Can you work these out from the drawing? Everything is in mm from the part's minimum corner. A direction names the side the tool comes from. Round coordinates to 2 decimals unless told otherwise and drop trailing zeros. Loops run counter-clockwise (first coordinate to the right, second up) from the corner with the lowest first, then second, coordinate; pieces in that order, holes last. Notation, with made-up numbers: (14.25, 82) -> (41.25, 82) arc R21 ccw to (41.25, 98) -> close; hole circle Ø7 at (64.5, 71.25). An arc over 180 degrees is marked (long way). One line per item, written item: value.
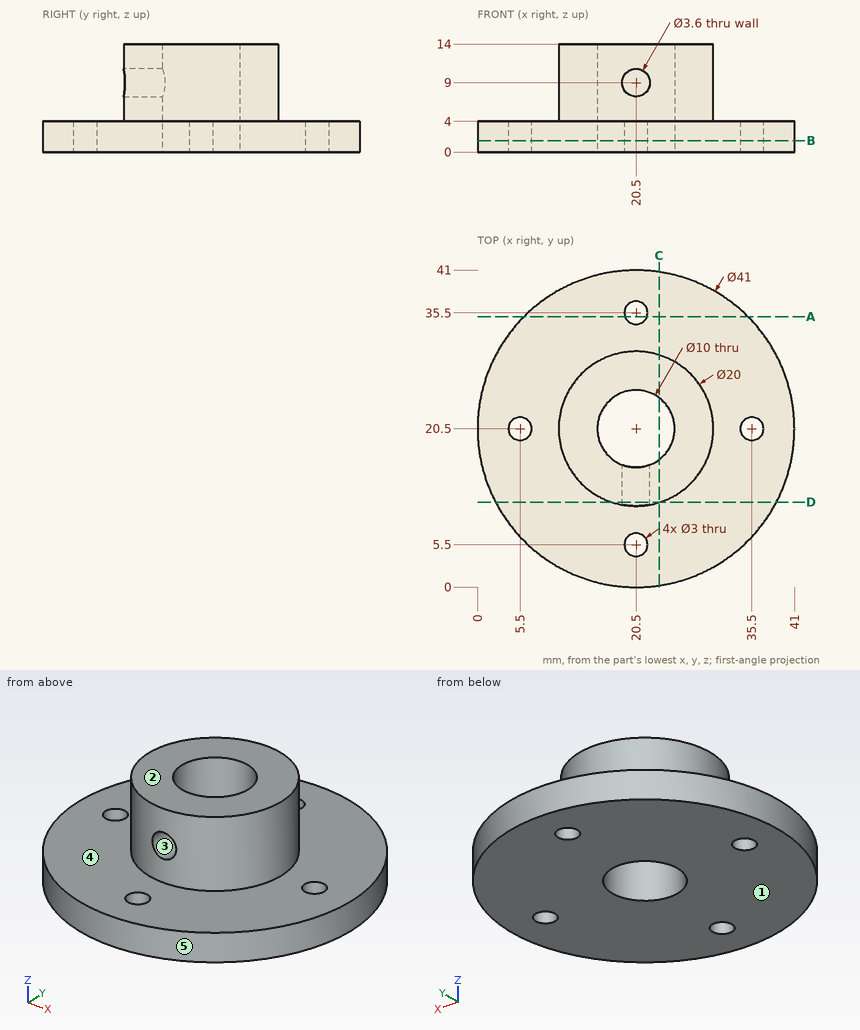
(1) Thinking about a two-plate mould opening in Z: for the marked faces 1, 2 and 3, which applies, released by +Z, released by -Z, zero draft, split by the parting line, or undercut?
Recorded:
face 1: released by -Z
face 2: released by +Z
face 3: undercut
(2) If we section it at B-B, the plane z = 1.5: Please give me the cut outline in (x, y).
Recorded:
outline: circle Ø41 at (20.5, 20.5); hole circle Ø3 at (5.5, 20.5); hole circle Ø10 at (20.5, 20.5); hole circle Ø3 at (20.5, 5.5); hole circle Ø3 at (20.5, 35.5); hole circle Ø3 at (35.5, 20.5)
(3) If we section it at C-C, the plane x = 23.5: Please give me the cut outline in (y, z).
Recorded:
outline: (0.22, 0) -> (16.5, 0) -> (16.5, 14) -> (10.96, 14) -> (10.96, 4) -> (0.22, 4) -> close; (24.5, 0) -> (40.78, 0) -> (40.78, 4) -> (30.04, 4) -> (30.04, 14) -> (24.5, 14) -> close
(4) For the marked faces 4 and 5, which set-ups out of +Z, -Z, +X, -X, +Y, -Y let a thin tool reach every point of the face, with its end or its side?
Recorded:
face 4: +Z
face 5: +Z, -Z
(5) I'm going to push flat-ended pins straight in: pin 1 Ø3 at (x, z) = (34, 2.5) entering from +Y; pin 2 Ø5 at (x, y) = (20.5, 5.5) entering from +Z; pin 3 Ø2.5 at (x, y) = (35.5, 20.5) entering from +Z; pin 4 Ø1 at (x, z) = (19.5, 6.5) entering from +Y. Where does each tip first touch, or does it pass through?
Recorded:
pin 1: y = 37.12
pin 2: z = 4
pin 3: through
pin 4: y = 30.49
(6) If we section it at D-D, the plane y = 11: Please give me the cut outline in (x, z), then the cut area to 3 significant figures.
Recorded:
outline: (2.33, 0) -> (38.67, 0) -> (38.67, 4) -> (23.62, 4) -> (23.62, 14) -> (17.38, 14) -> (17.38, 4) -> (2.33, 4) -> close; hole circle Ø3.6 at (20.5, 9)
area: 198 mm²
(7) If we section it at A-A, the plane y = 35: Please give me the cut outline in (x, z), then the cut area to 3 significant figures.
Recorded:
outline: (6.01, 0) -> (19.09, 0) -> (19.09, 4) -> (6.01, 4) -> close; (21.91, 0) -> (34.99, 0) -> (34.99, 4) -> (21.91, 4) -> close
area: 105 mm²
(8) If I drill on L1, parallel to Y at x = 20.5, z = 1.7; L2, parallel to Z at x = 2, y = 21.5; L3, parallel to Y at x = 36, z = 2, over which ranges is the centre line in solid material (lowest first)?
Recorded:
L1: 0 to 4, 7 to 15.5, 25.5 to 34, 37 to 41
L2: 0 to 4
L3: 7.08 to 19.09, 21.91 to 33.92
